Can you work these out from the model? Positions are in its coordinate system, mm. A direction names the side the tool comes from. Coordinates: 2 decimals unless noted, no trailing zeros. Order: outer loops, then holes, each group sorted by start corner. A loop starts at its lowest first (then second) coordinate and runs counter-clockwise, first axis right, second up. Notation, with made-up numbers: (30.25, 54.5) - (82.25, 54.5) arc R17 ccw to (82.25, 77.5) - close; hole circle Ø7 at (88, -37.5). An arc over 180 degrees is marked (long way). Return JSON: item names as keys, results as strings. Group by question number.
1) If we mould it in two halves opening along X, with no side actions, what happens to faces 3 (the face through (-7, -20, 6)), 4 (the face through (0, 0, 54.5)), 5 (the face through (-29.97, -1.32, 33.61)), 6 (the face through (10.382, -19.961, 58.302))? For each: pulls with the +X half, pulls with the -X half, needs draft (parallel to the pull), parting line crosses it, or undercut.
2) If I drill on line 1 along Y through (x, z) = (0, 56); line 2 along Z through (x, y) = (-23, 13.5); line 3 along Z through (x, y) = (-18, -6), over which ranges is the centre line in solid material (lowest first)?
3) Imagine slicing it at D-D (z = 29). Write out the boundary of the cut face in (x, y).
4) For pin 1 Ø1 at (y, z) = (10.5, 30.5) entering from -X; pin 2 Ø1 at (x, z) = (2.5, 30) entering from -Y; pin 3 Ø12 at (x, z) = (-6.5, 14) entering from -Y; pin 4 Ø5 at (x, y) = (-21, -1.5) entering from +Z, each with a flat end and sliding along its axis, tell me the tip position at first contact or that it passes through.
5) Which directions (+Z, -Z, +X, -X, +Y, -Y) give clear straight access to the entire face, cutting with the end or side of a thin tool? Please do faces 1 (the face through (19.99, -6.29, 5.62)), 2 (the face through (4.3, 22.4, 62)).
6) Imagine slicing it at A-A (z = 57). Write out the boundary of the cut face in (x, y), and give its area (3 significant figures).
7) Imagine slicing it at B-B (x = 0). Write out the boundary of the cut face in (y, z), and give its area (3 significant figures).
Autodesk Inventor part; units mm, degrees
ref_plane "YZ Plane" through (0, 0, 0) normal (1, 0, 0) x (0, 1, 0)
ref_plane "XZ Plane" through (0, 0, 0) normal (0, 1, 0) x (-1, 0, 0)
ref_plane "XY Plane" through (0, 0, 0) normal (0, 0, 1) x (1, 0, 0)
sketch "Sketch1" plane through (0, 0, 0) normal (0, 0, 1) x (1, 0, 0)
  circle A0 centre (0, 0) radius 23
  dimension "d0" = 46
extrude "Extrusion1" add sketch "Sketch1" along normal blind 6 draft -20
sketch "Sketch2" plane through (0, 0, 6) normal (0, 0, 1) x (1, 0, 0)
  circle A0 centre (0, 0) radius 30
  dimension "d3" = 60
extrude "Extrusion2" add sketch "Sketch2" along normal blind 56
sketch "Sketch3" plane through (0, 0, 62) normal (0, 0, 1) x (1, 0, 0)
  circle A0 centre (0, 0) radius 22.5
  dimension "d6" = 45
extrude "Extrusion3" cut sketch "Sketch3" against normal blind 7.5
properties part number "olympusTubeLens" material "Aluminum 6061"
Calculated:
{
 "1": {"face 3": "needs draft", "face 4": "undercut", "face 5": "parting line crosses it", "face 6": "undercut"},
 "2": {"line 1": "-30 to -22.5, 22.5 to 30", "line 2": "6 to 62", "line 3": "0 to 54.5"},
 "3": {"outline": "circle Ø60 at (0, 0)"},
 "4": {"pin 1": "x = -28.28", "pin 2": "y = -29.93", "pin 3": "y = -30", "pin 4": "z = 62"},
 "5": {"face 1": "none", "face 2": "+Z, +X, -X, +Y, -Y"},
 "6": {"outline": "circle Ø60 at (0, 0); hole circle Ø45 at (0, 0)", "area": "1,240 mm2"},
 "7": {"outline": "(-30, 6) - (-20.82, 6) - (-23, 0) - (23, 0) - (20.82, 6) - (30, 6) - (30, 62) - (22.5, 62) - (22.5, 54.5) - (-22.5, 54.5) - (-22.5, 62) - (-30, 62) - close", "area": "3,290 mm2"}
}
